from build123d import *

# Parameters (mm, degrees)
EXTRUDE_1_DEPTH              = 7
CUT_EXTRUDE_1_DEPTH          = 4
HOLE_WIZARD_M3_1_D           = 3.4
HOLE_WIZARD_M3_1_DEPTH       = 7.5
HOLE_WIZARD_M3_1_CSINK_D     = 6.72
HOLE_WIZARD_M3_1_CSINK_ANGLE = 90
HOLE_WIZARD_M3_1_TIP         = 1.021463052
HOLE_WIZARD_1_D              = 4.15
CUT_EXTRUDE_2_DEPTH          = 4


with BuildPart() as part:
    # 草图1 → 凸台-拉伸1 (new body)
    with BuildSketch(Plane.XY):
        with BuildLine():
            Line((0, 5), (10, 5))
            ThreePointArc((10, 5), (15, 0), (10, -5))
            Line((10, -5), (0, -5))
            ThreePointArc((0, -5), (-5, 0), (0, 5))
        make_face()
    extrude(amount=EXTRUDE_1_DEPTH)

    # 草图2 → 切除-拉伸1 (cut)
    with BuildSketch(Plane.XY.offset(7)):
        with BuildLine():
            Line((1.5, 2), (-1.5, 2))
            ThreePointArc((-1.5, 2), (-2.5, 0), (-1.5, -2))
            Line((-1.5, -2), (1.5, -2))
            ThreePointArc((1.5, -2), (2.236067977, -1.118033989), (2.5, 0))
            ThreePointArc((2.5, 0), (2.236067977, 1.118033989), (1.5, 2))
        make_face()
    extrude(amount=-CUT_EXTRUDE_1_DEPTH, mode=Mode.SUBTRACT)

    # M3 六角凹锥坑螺钉的锥形沉头孔1
    with Locations(Plane(origin=(0, 0, 0), x_dir=(-1, 0, 0), z_dir=(0, 0, -1))):
        with Locations((0, 0)):
            CounterSinkHole(HOLE_WIZARD_M3_1_D / 2, HOLE_WIZARD_M3_1_CSINK_D / 2, depth=HOLE_WIZARD_M3_1_DEPTH, counter_sink_angle=HOLE_WIZARD_M3_1_CSINK_ANGLE)
            with Locations((0, 0, -(HOLE_WIZARD_M3_1_DEPTH + HOLE_WIZARD_M3_1_TIP / 2))):  # 118° drill point
                Cone(0, HOLE_WIZARD_M3_1_D / 2, HOLE_WIZARD_M3_1_TIP, mode=Mode.SUBTRACT)

    # 孔1 (through all)
    with Locations(Plane(origin=(0, 0, 0), x_dir=(-1, 0, 0), z_dir=(0, 0, -1))):
        with Locations((-10, 0)):
            Hole(HOLE_WIZARD_1_D / 2)

    # 草图7 → 切除-拉伸2 (cut)
    with BuildSketch(Plane.XY.offset(7)):
        Polygon((8.325684219, -2.9), (11.674315781, -2.9), (13.348631561, 0), (11.674315781, 2.9), (8.325684219, 2.9), (6.651368439, 0), align=None)
    extrude(amount=-CUT_EXTRUDE_2_DEPTH, mode=Mode.SUBTRACT)


solid = part.part
CAD build for the part. Positions are in the model's coordinates, mm. A direction names the side the tool comes from. Coordinates: 2 decimals unless noted, no trailing zeros. Loops run counter-clockwise (first coordinate to the right, second up) from the corner with the lowest first, then second, coordinate; pieces in that order, holes last. Notation, with made-up numbers: (11.25, 84.5) -> (65.25, 84.5) arc R15 ccw to (65.25, 93.5) -> close; hole circle Ø4 at (-23.75, 31). An arc over 180 degrees is marked (long way). One line per item, written item: value.
1. Slice it at A-A on z = 4.75. Write the cut outline in (x, y), and give its area (3 significant figures).
Answers:
outline: (0, -5) -> (10, -5) arc R5 ccw to (10, 5) -> (0, 5) arc R5 ccw to start; hole (-1.5, -2) -> (1.5, -2) arc R2.5 ccw to (1.5, 2) -> (-1.5, 2) arc R2.5 ccw to start; hole (6.65, 0) -> (8.33, -2.9) -> (11.67, -2.9) -> (13.35, 0) -> (11.67, 2.9) -> (8.33, 2.9) -> close
area: 132 mm^2
2. Drill centre lines: line 1 (Y direction, x = 10, z = 1.5) (3 decimals); line 2 (Y direction, x = 0, z = 2.5); line 3 (X direction, y = -2.75, z = 6.5). Where is each one in solid material? Low to high. Write a range as [from, to].
Answers:
line 1: y = [-5, -2.075], [2.075, 5]
line 2: y = [-5, -1.7], [1.7, 5]
line 3: x = [-4.18, 8.24], [11.76, 14.18]
3. Flat gauge pins, fed straight in: P1, Ø3.5, axis at x = 10, y = 0, coming from the -Z side; P2, Ø4, axis at y = 2.5, z = 3, coming from the +X side. Where does each tip first touch, or does it go through?
Answers:
P1: passes through
P2: stops at x = 14.97
4. Slice it at D-D on y = -0.75. Give the number of separate pieces and of enclosed holes in the cut face, and give its area (3 significant figures).
Answers:
separate pieces: 3
enclosed holes: 0
area: 73.1 mm^2
5. Slice it at C-C on x = 13. Write the cut outline in (y, z).
Answers:
outline: (-4, 0) -> (4, 0) -> (4, 7) -> (0.6, 7) -> (0.6, 3) -> (-0.6, 3) -> (-0.6, 7) -> (-4, 7) -> close
6. Slice it at B-B on z = 0.5. Write the cut outline in (x, y) (3 decimals), and give its area (3 significant figures).
Answers:
outline: (0, -5) -> (10, -5) arc R5 ccw to (10, 5) -> (0, 5) arc R5 ccw to start; hole circle Ø5.72 at (0, 0); hole circle Ø4.15 at (10, 0)
area: 139 mm^2
7. Which spindle directions (+Z, -Z, +X, -X, +Y, -Y) get a long thin tool onto all of the face, cutting with end or side? Do faces 4 (the face through (-2.5, 0, 5)), 5 (the face through (-0.37, -1.66, 2.34)). Say none if no direction does.
Answers:
face 4: +Z
face 5: +Z, -Z
8. Pull direction X, two halves, no side cores. Call faces 1 (the face through (-5, 0, 3)), 2 (the face through (5, -5, 3)), 3 (the face through (12.5, -1.47, 5.03)): pulls with the +X half, pulls with the -X half, needs draft (parallel to the pull), parting line crosses it, or undercut.
Answers:
face 1: pulls with the -X half
face 2: needs draft
face 3: undercut
